Read the model definition and answer for the solid it produces. Units are mm, in the model's axes. A direction names the side the tool comes from. Coordinates: 2 decimals unless noted, no trailing zeros. Write each loop counter-clockwise with the first axis right and the second up, starting at its lowest first coordinate (ties: lowest second). Pieces come first, ordered by that corner, then holes.
from build123d import *

# Parameters (mm, degrees)
SKETCH2_W           = 200
SKETCH2_H           = 40
BOSS_EXTRUDE1_DEPTH = 40
SKETCH3_R           = 18
BOSS_EXTRUDE2_DEPTH = 10
SKETCH4_R           = 5
CUT_EXTRUDE1_DEPTH  = 51
SKETCH5_R           = 3.5
CUT_EXTRUDE2_DEPTH  = 51


with BuildPart() as part:
    # Sketch2 → Boss-Extrude1 (new body)
    with BuildSketch(Plane(origin=(0, 0, 0), x_dir=(1, 0, 0), z_dir=(0, 1, 0))):
        with Locations((100, 20)):
            Rectangle(SKETCH2_W, SKETCH2_H)
    extrude(amount=BOSS_EXTRUDE1_DEPTH)

    # Sketch3 → Boss-Extrude2 (add)
    with BuildSketch(Plane(origin=(0, 0, -40), x_dir=(-1, 0, 0), z_dir=(0, 0, -1))):
        with Locations(Location((-100, 30, 0), (0, 0, 146.251011404))):
            Circle(SKETCH3_R)
    extrude(amount=BOSS_EXTRUDE2_DEPTH)

    # Sketch4 → Cut-Extrude1 (cut)
    with BuildSketch(Plane(origin=(0, 0, -50), x_dir=(-1, 0, 0), z_dir=(0, 0, -1))):
        with Locations((-100, 30)):
            Circle(SKETCH4_R)
    extrude(amount=-CUT_EXTRUDE1_DEPTH, mode=Mode.SUBTRACT)

    # Sketch5 → Cut-Extrude2 (cut)
    with BuildSketch(Plane(origin=(0, 0, -50), x_dir=(-1, 0, 0), z_dir=(0, 0, -1))):
        with Locations((-77.5, 30)):
            Circle(SKETCH5_R)
        with Locations((-122.5, 30)):
            Circle(SKETCH5_R)
    extrude(amount=-CUT_EXTRUDE2_DEPTH, mode=Mode.SUBTRACT)


solid = part.part
Item 1: Determine the mould class of faces 3 (the flat face through (0, 20, -20)), 4 (the cylindrical face through (95.381, 28.085, -25.35)), 5 (the cylindrical face through (82.04, 31.17, -44.93)), 6 (the flat face through (101, 35.2, -50)) for opening direction X: +X half, -X half, draft (parallel to the pull), parting line (faces both ways), or undercut.
Item 2: The part is cut by section A-A (y = 30). Give the vertices of the cut face in (x, z), and give its area (3 significant figures).
Item 3: The part is cut by section C-C (z = -3.5). Give the vertices of the cut face in (x, y), and give its area (3 significant figures).
Item 4: The part is cut by section B-B (x = 77.5). Give the vertices of the cut face in (y, z).
Item 5: Find the intervals of material crossed by probe 1 along Y at (x, z) = (122.5, -26.5); probe 2 along Y at (x, z) = (12.5, -39); probe 3 along Y at (x, z) = (100.5, -2.5), in increasing order.
Item 6: For faces 1 (the flat face through (99, 20, 0)), 2 (the flat face through (101, 44, -40)), determine the directions among +Z, -Z, +X, -X, +Y, -Y from which every point of the face is accessible in a straight line to the end or side of a thin tool.
Item 7: The part is cut by section D-D (x = 100). Give the vertices of the cut face in (y, z).
Item 8: Given pin 1 (8 mm diameter, centred on x = 100, y = 30, fed in from +Z); pin 2 (1 mm diameter, centred on x = 121.5, z = -18, fed in from +Y); pin 3 (12 mm diameter, centred on x = 164.5, y = 41.5, fed in from -Z), each flat-ended and moving along its own axis, determine where each tip first touches the part or whether it passes through.
Answer:
1. face 3: -X half
1. face 4: undercut
1. face 5: parting line
1. face 6: draft
2. outline: (0, -40) - (74, -40) - (74, 0) - (0, 0) - close; (81, -40) - (82, -40) - (82, -50) - (95, -50) - (95, 0) - (81, 0) - close; (105, -50) - (118, -50) - (118, -40) - (119, -40) - (119, 0) - (105, 0) - close; (126, -40) - (200, -40) - (200, 0) - (126, 0) - close
2. area: 7,300 mm2
3. outline: (0, 0) - (200, 0) - (200, 40) - (0, 40) - close; hole circle Ø7 at (77.5, 30); hole circle Ø10 at (100, 30); hole circle Ø7 at (122.5, 30)
3. area: 7,840 mm2
4. outline: (0, -40) - (26.5, -40) - (26.5, 0) - (0, 0) - close; (33.5, -40) - (40, -40) - (40, 0) - (33.5, 0) - close
5. probe 1: y = 0 to 26.5, 33.5 to 40
5. probe 2: y = 0 to 40
5. probe 3: y = 0 to 25.03, 34.97 to 40
6. face 1: +Z, +X, -X, +Y, -Y
6. face 2: +Z, +X, -X, +Y
7. outline: (0, -40) - (12, -40) - (12, -50) - (25, -50) - (25, 0) - (0, 0) - close; (35, -50) - (48, -50) - (48, -40) - (40, -40) - (40, 0) - (35, 0) - close
8. pin 1: passes through
8. pin 2: stops at y = 40
8. pin 3: stops at z = -40
